Verification items for the finished model (mm, model axes). Face numbers are marked on the shaded views. Round coordinates to 2 decimals unless told otherwise and drop trailing zeros. Loops run counter-clockwise (first coordinate to the right, second up) from the corner with the lowest first, then second, coordinate; pieces in that order, holes last. Notation, with made-up numbers: (89, 13.5) -> (99, 13.5) arc R17 cw to (99, 22.5) -> close; hole circle Ø1 at (18.25, 49.5). An arc over 180 degrees is marked (long way). Write item = value, one per line.
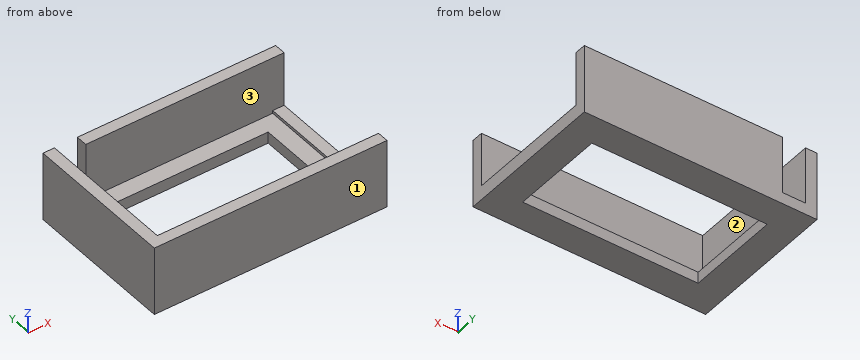
```python
from build123d import *

# Parameters (mm, degrees)
ESQUISSE1_W             = 20.32
ESQUISSE1_H             = 13.2
BOSS_EXTRU_1_DEPTH      = 6
ESQUISSE2_W             = 18.32
ESQUISSE2_H             = 11.2
ENL_V_MAT_EXTRU_1_DEPTH = 5
ESQUISSE3_W             = 2
ESQUISSE3_H             = 1
ENL_V_MAT_EXTRU_2_DEPTH = 5
ESQUISSE4_W             = 15.32
ESQUISSE4_H             = 8.2
ENL_V_MAT_EXTRU_3_DEPTH = 25.741511676
ESQUISSE6_W             = 1
ESQUISSE6_H             = 11.2
ENL_V_MAT_EXTRU_4_DEPTH = 4.75


with BuildPart() as part:
    # Esquisse1 → Boss.-Extru.1 (new body)
    with BuildSketch(Plane.XY):
        with Locations((10.16, 6.6)):
            Rectangle(ESQUISSE1_W, ESQUISSE1_H)
    extrude(amount=BOSS_EXTRU_1_DEPTH)

    # Esquisse2 → Enlèv. mat.-Extru.1 (cut)
    with BuildSketch(Plane.XY.offset(6)):
        with Locations((10.16, 6.6)):
            Rectangle(ESQUISSE2_W, ESQUISSE2_H)
    extrude(amount=-ENL_V_MAT_EXTRU_1_DEPTH, mode=Mode.SUBTRACT)

    # Esquisse3 → Enlèv. mat.-Extru.2 (cut)
    with BuildSketch(Plane.XY.offset(6)):
        with Locations((2, 12.7)):
            Rectangle(ESQUISSE3_W, ESQUISSE3_H)
    extrude(amount=-ENL_V_MAT_EXTRU_2_DEPTH, mode=Mode.SUBTRACT)

    # Esquisse4 → Enlèv. mat.-Extru.3 (cut, through all)
    with BuildSketch(Plane.XY.offset(1)):
        with Locations((10.16, 6.6)):
            Rectangle(ESQUISSE4_W, ESQUISSE4_H)
    extrude(amount=-ENL_V_MAT_EXTRU_3_DEPTH, mode=Mode.SUBTRACT)

    # Esquisse6 → Enlèv. mat.-Extru.4 (cut)
    with BuildSketch(Plane.XY.offset(6)):
        with Locations((19.82, 6.6)):
            Rectangle(ESQUISSE6_W, ESQUISSE6_H)
    extrude(amount=-ENL_V_MAT_EXTRU_4_DEPTH, mode=Mode.SUBTRACT)


solid = part.part
```
(1) Sectioned sample at C-C, the plane y = 10.5. Record the cut outline in (x, z), and give its area (4 significant figures).
Filled sheet:
outline = (0, 0) -> (2.5, 0) -> (2.5, 1) -> (1, 1) -> (1, 6) -> (0, 6) -> close; (17.82, 0) -> (20.32, 0) -> (20.32, 1.25) -> (19.32, 1.25) -> (19.32, 1) -> (17.82, 1) -> close
area = 10.25 mm2
(2) Draft check along Y on the marked faces 1, 2 and 3. Enter one of: released by +Y, released by -Y, zero draft, split by the parting line, or undercut.
Filled sheet:
face_1 = released by -Y
face_2 = zero draft
face_3 = undercut
(3) Material ranges on probe 1 along Y at (x, z) = (11.75, 1.7); probe 2 along X at (y, z) = (12.75, 4.2); probe 3 along X at (y, z) = (6.25, 0.9), recorded low to high. Write a range as from..to.
Filled sheet:
probe_1 = 0..1, 12.2..13.2
probe_2 = 0..1, 3..20.32
probe_3 = 0..2.5, 17.82..20.32
(4) Sectioned sample at A-A, the plane z = 2.5. Record the cut outline in (x, y), and give its area (3 significant figures).
Filled sheet:
outline = (0, 0) -> (20.32, 0) -> (20.32, 1) -> (1, 1) -> (1, 13.2) -> (0, 13.2) -> close; (3, 12.2) -> (20.32, 12.2) -> (20.32, 13.2) -> (3, 13.2) -> close
area = 49.8 mm2
(5) Sectioned sample at D-D, the plane z = 0.55. Record the cut outline in (x, y).
Filled sheet:
outline = (0, 0) -> (20.32, 0) -> (20.32, 13.2) -> (0, 13.2) -> close; hole (2.5, 2.5) -> (17.82, 2.5) -> (17.82, 10.7) -> (2.5, 10.7) -> close
(6) Sectioned sample at B-B, the plane x = 10.25. Record the cut outline in (y, z), and give its area (3 significant figures).
Filled sheet:
outline = (0, 0) -> (2.5, 0) -> (2.5, 1) -> (1, 1) -> (1, 6) -> (0, 6) -> close; (10.7, 0) -> (13.2, 0) -> (13.2, 6) -> (12.2, 6) -> (12.2, 1) -> (10.7, 1) -> close
area = 15.0 mm2
(7) Go/stop test with flat-tipped pins: pin 1 Ø0.8 at (x, z) = (10, 0.5) entering from -Y; pin 2 Ø0.5 at (x, y) = (20, 7.5) entering from +Z. Record where each tip stops, or that it passes through.
Filled sheet:
pin_1 = 0
pin_2 = 1.25
